The model under review builds one solid part; all positions refer to its coordinate system, in mm. A direction names the side the tool comes from. Give positions to 0.01 mm unless a question says otherwise; leave off trailing zeros. Loops run counter-clockwise (first coordinate to the right, second up) from the corner with the lowest first, then second, coordinate; pieces in that order, holes last. Notation, with made-up numbers: (75, 0) - (87, 0) arc R9 cw to (87, 15) - close; hole circle Ø7 at (66, 23). An arc over 180 degrees is marked (long way). Return JSON: item names as keys, results as strings. Group by question number.
```python
from build123d import *

# Parameters (mm, degrees)
BOSS_EXTRUDE1_DEPTH = 0.1
BOSS_EXTRUDE2_DEPTH = 0.3
BOSS_EXTRUDE3_DEPTH = 1.6
BOSS_EXTRUDE4_DEPTH = 1
BOSS_EXTRUDE6_DEPTH = 2


with BuildPart() as part:
    # Sketch1 → Boss-Extrude1 (new body)
    with BuildSketch(Plane(origin=(0, 0, 0), x_dir=(1, 0, 0), z_dir=(0, 1, 0))):
        Polygon((-10.891797249, 26.577808825), (-5.79351947, 9.149986826), (-2.397224373, 3.489407839), (5.640466214, 5.66196227), (-0.734212813, 29.279724171), align=None)
    extrude(amount=-BOSS_EXTRUDE1_DEPTH)



with BuildPart() as body_2:
    # Sketch1_4 → Boss-Extrude2 (new body)
    with BuildSketch(Plane(origin=(0, 0, 0), x_dir=(1, 0, 0), z_dir=(0, 1, 0))):
        Polygon((11.001219022, 9.275344539), (7.705525211, 33.438949507), (18.007446345, 34.7772024), (21.345127352, 10.801402821), align=None)
    extrude(amount=-BOSS_EXTRUDE2_DEPTH)


with BuildPart() as body_3:
    # Sketch1_6 → Boss-Extrude3 (new body)
    with BuildSketch(Plane(origin=(0, 0, 0), x_dir=(1, 0, 0), z_dir=(0, 1, 0))):
        Polygon((33.233450435, 10.417934204), (34.248462201, 34.6301789), (23.994142325, 35.215869617), (23.110432029, 10.99610324), align=None)
    extrude(amount=-BOSS_EXTRUDE3_DEPTH)


with BuildPart() as body_4:
    # Sketch1_7 → Boss-Extrude4 (new body)
    with BuildSketch(Plane(origin=(0, 0, 0), x_dir=(1, 0, 0), z_dir=(0, 1, 0))):
        Polygon((34.143873473, 5.198308151), (38.309825185, 29.363057326), (48.452043785, 27.653721075), (44.159317146, 3.708440275), align=None)
    extrude(amount=-BOSS_EXTRUDE4_DEPTH)


with BuildPart() as part_1:
    add(part.part)

    add(body_2.part)  # Boss-Extrude6 merges body 2

    add(body_3.part)  # Boss-Extrude6 merges body 3

    add(body_4.part)  # Boss-Extrude6 merges body 4
    # Sketch1_9 → Boss-Extrude6 (add)
    with BuildSketch(Plane(origin=(0, 0, 0), x_dir=(1, 0, 0), z_dir=(0, 1, 0))):
        Polygon((-10.986197156, 29.721735633), (-16.549013322, 27.076085928), (-0.25286222, -0.084584113), (2.807938166, 0.939274203), (23.783364855, 4.743803832), (44.5054493, 1.124608783), (47.119494483, 0.837420224), (49.023338551, 5.65160383), (45.570660298, 7.575242468), (51.160151479, 17.793063144), (59.478406067, 27.913224514), (48.433689461, 31.007653737), (39.469998377, 32.102859377), (37.111434986, 37.337196557), (33.923134788, 37.655423442), (24.762205898, 38.01292185), (16.732720281, 37.515854171), (8.013100705, 36.602302747), (-2.397224373, 32.120681941), align=None)
    extrude(amount=BOSS_EXTRUDE6_DEPTH)


solid = part_1.part
```
1) We need section A-A, the plane y = 0.95. Write out the cut boundary in (x, z).
2) For pin 1 Ø11 at (x, z) = (13.5, -19) entering from -Y; pin 2 Ø2 at (x, y) = (21, 1.5) entering from -Z; pin 3 Ø13 at (x, z) = (-2, -20.5) entering from -Y; pin 4 Ø15.5 at (x, z) = (39.5, -16) entering from -Y, all flat-tipped, find the tip position at first contact; note any pin that passes through.
3) We need section D-D, the plane x = 50. Write out the cut boundary in (y, z), plus the area to 3 significant figures.
4) To check wall thickness, follow line 1 (X direction, y = -0.15, z = -12.5); line 2 (X direction, y = -0.2, z = -27); line 3 (Y direction, x = 43.5, z = -5.5). State the ranges of each line that lie inside material, in increasing order.
5) Tool access review of faces 4 (the face through (45.794, 0.986, -0.983)), 5 (the face through (21, 0, -20)), 6 (the face through (47.32, 0.99, -6.6)): name each direction out of +Z, -Z, +X, -X, +Y, -Y from which nothing blocks a thin tool from reaching the whole face with its end or side.
6) We need section C-C, the plane x = 32. Write out the cut boundary in (y, z).
7) Draft analysis for pull direction X (two halves, no side actions). For faces 1 (the face through (20.804, 0.986, -37.768)), 2 (the face through (23.56, -0.79, -23.28)), 3 (the face through (48.326, 0.986, -12.613)), state which applies: +X half, -X half, draft (parallel to the pull), parting line (faces both ways), or undercut.
8) We need section B-B, the plane z = -16.5. Write out the cut boundary in (x, y), plus the area to 3 significant figures.
Findings:
{
 "1": {"outline": "(-16.55, -27.08) - (-10.99, -29.72) - (-2.4, -32.12) - (8.01, -36.6) - (16.73, -37.52) - (24.76, -38.01) - (33.92, -37.66) - (37.11, -37.34) - (39.47, -32.1) - (48.43, -31.01) - (59.48, -27.91) - (51.16, -17.79) - (45.57, -7.58) - (49.02, -5.65) - (47.12, -0.84) - (44.51, -1.12) - (23.78, -4.74) - (2.81, -0.94) - (-0.25, 0.08) - close"},
 "2": {"pin 1": "stops at y = -0.3", "pin 2": "stops at z = -37.84", "pin 3": "stops at y = -0.1", "pin 4": "stops at y = -1.6"},
 "3": {"outline": "(0, -30.57) - (2, -30.57) - (2, -15.67) - (0, -15.67) - close", "area": "29.8 mm^2"},
 "4": {"line 1": "x = 10.56 to 21.11, 23.17 to 33.32, 35.4 to 45.74", "line 2": "x = 8.58 to 19.09, 23.69 to 33.93, 37.9 to 48.33", "line 3": "y = -1 to 2"},
 "5": {"face 4": "+Z, +Y, -Y", "face 5": "-Y", "face 6": "+X, +Y, -Y"},
 "6": {"outline": "(-1.6, -34.76) - (0, -34.76) - (0, -37.73) - (2, -37.73) - (2, -3.31) - (0, -3.31) - (0, -10.49) - (-1.6, -10.49) - close"},
 "7": {"face 1": "-X half", "face 2": "undercut", "face 3": "+X half"},
 "8": {"outline": "(-10.2, 0) - (-7.94, 0) - (-7.94, -0.1) - (2.72, -0.1) - (2.72, 0) - (10.02, 0) - (10.02, -0.3) - (20.55, -0.3) - (20.55, 0) - (23.31, 0) - (23.31, -1.6) - (33.49, -1.6) - (33.49, 0) - (36.09, 0) - (36.09, -1) - (46.45, -1) - (46.45, 0) - (50.45, 0) - (50.45, 2) - (-10.2, 2) - close", "area": "152 mm^2"}
}
